```python
from build123d import *

# Parameters (mm, degrees)
BOSS_EXTRUDE1_DEPTH = 2
SKETCH1_3_W         = 10
SKETCH1_3_H         = 4.75
BOSS_EXTRUDE2_DEPTH = 12.7
BOSS_EXTRUDE3_START = 12.7
SKETCH3_W           = 11.9
SKETCH3_H           = 4.75
SKETCH3_W_2         = 10.75
BOSS_EXTRUDE3_DEPTH = 12.7
BOSS_EXTRUDE4_START = 25.4
SKETCH3_3_W         = 11.9
SKETCH3_3_H         = 4.75
SKETCH3_3_W_2       = 10.75
SKETCH3_3_W_3       = 1.15
BOSS_EXTRUDE4_DEPTH = 2
CUT_EXTRUDE1_START  = -1.1
SKETCH2_R           = 1.6
CUT_EXTRUDE1_DEPTH  = 8
CUT_EXTRUDE2_START  = 3.1
SKETCH2_3_R         = 1.6
CUT_EXTRUDE2_DEPTH  = 8
BOSS_EXTRUDE5_START = 10
SKETCH1_4_R         = 2.075
BOSS_EXTRUDE5_DEPTH = 10
FILLET1_R           = 5
CUT_EXTRUDE3_START  = 12.7
SKETCH5_W           = 14.55
SKETCH5_H           = 4.75
CUT_EXTRUDE3_DEPTH  = 2
CUT_EXTRUDE4_START  = 12.7
SKETCH6_W           = 7.7
SKETCH6_H           = 4.75
CUT_EXTRUDE4_DEPTH  = 4


with BuildPart() as part:
    # Sketch1 → Boss-Extrude1 (new body)
    with BuildSketch(Plane(origin=(0, 0, 0), x_dir=(1, 0, 0), z_dir=(0, 1, 0))):
        Polygon((-1.1, 16.25), (-1.1, -16.25), (8.9, -16.25), (8.9, -11.5), (17.65, -11.5), (17.65, 16.25), align=None)
    extrude(amount=-BOSS_EXTRUDE1_DEPTH)

    # Sketch1<3> → Boss-Extrude2 (add)
    with BuildSketch(Plane(origin=(0, 0, 0), x_dir=(1, 0, 0), z_dir=(0, 1, 0))):
        Polygon((6.45, 16.25), (-1.1, 16.25), (-1.1, 11.5), (17.65, 11.5), (17.65, 16.25), align=None)
        with Locations((3.9, -13.875)):
            Rectangle(SKETCH1_3_W, SKETCH1_3_H)
    extrude(amount=BOSS_EXTRUDE2_DEPTH)

    # Sketch3 → Boss-Extrude3 (add)
    with BuildSketch(Plane(origin=(0, 0, 0), x_dir=(1, 0, 0), z_dir=(0, 1, 0)).offset(BOSS_EXTRUDE3_START)):
        with Locations((-2.85, 13.875)):
            Rectangle(SKETCH3_W, SKETCH3_H)
        with Locations((-2.275, -13.875)):
            Rectangle(SKETCH3_W_2, SKETCH3_H)
    extrude(amount=BOSS_EXTRUDE3_DEPTH)

    # Sketch3<3> → Boss-Extrude4 (add)
    with BuildSketch(Plane(origin=(0, 0, 0), x_dir=(1, 0, 0), z_dir=(0, 1, 0)).offset(BOSS_EXTRUDE4_START)):
        with Locations((-2.85, 13.875)):
            Rectangle(SKETCH3_3_W, SKETCH3_3_H)
        Polygon((3.1, -11.5), (3.1, 11.5), (-8.8, 11.5), (-8.8, -11.5), (-7.65, -11.5), align=None)
        with Locations((-2.275, -13.875)):
            Rectangle(SKETCH3_3_W_2, SKETCH3_3_H)
        with Locations((-8.225, -13.875)):
            Rectangle(SKETCH3_3_W_3, SKETCH3_3_H)
    extrude(amount=BOSS_EXTRUDE4_DEPTH)

    # Sketch2 → Cut-Extrude1 (cut)
    with BuildSketch(Plane(origin=(0, 0, 0), x_dir=(0, 0, -1), z_dir=(1, 0, 0)).offset(CUT_EXTRUDE1_START)):
        with Locations(Location((-13.7, 6.45, 0), (0, 0, 180))):
            Circle(SKETCH2_R)
        with Locations(Location((13.7, 6.45, 0), (0, 0, 180))):
            Circle(SKETCH2_R)
    extrude(amount=CUT_EXTRUDE1_DEPTH, mode=Mode.SUBTRACT)

    # Sketch2<3> → Cut-Extrude2 (cut)
    with BuildSketch(Plane(origin=(0, 0, 0), x_dir=(0, 0, -1), z_dir=(1, 0, 0)).offset(CUT_EXTRUDE2_START)):
        with Locations(Location((13.7, 19.15, 0), (0, 0, 180))):
            Circle(SKETCH2_3_R)
        with Locations(Location((-13.7, 19.15, 0), (0, 0, 180))):
            Circle(SKETCH2_3_R)
    extrude(amount=-CUT_EXTRUDE2_DEPTH, mode=Mode.SUBTRACT)

    # Sketch1<4> → Boss-Extrude5 (add)
    # profile 1 of 2: a face of its own
    with BuildSketch(Plane(origin=(0, 0, 0), x_dir=(1, 0, 0), z_dir=(0, 1, 0)).offset(BOSS_EXTRUDE5_START)):
        Polygon((-1.25, 16.25), (-1.1, 16.25), (6.45, 16.25), (6.45, 23.05), (-1.25, 23.05), align=None)
        with Locations(Location((2.6, 19.85, 0), (0, 0, 270))):
            Circle(SKETCH1_4_R, mode=Mode.SUBTRACT)
    # profile 2 of 2: a face of its own
    with BuildSketch(Plane(origin=(0, 0, 0), x_dir=(1, 0, 0), z_dir=(0, 1, 0)).offset(BOSS_EXTRUDE5_START)):
        Polygon((-3.95, -23.05), (-3.95, -16.25), (-8.8, -16.25), (-11.65, -16.25), (-11.65, -23.05), align=None)
        with Locations(Location((-7.8, -19.85, 0), (0, 0, 270))):
            Circle(SKETCH1_4_R, mode=Mode.SUBTRACT)
    extrude(amount=BOSS_EXTRUDE5_DEPTH)

    # Fillet1
    fillet1_edges = [part.edges().sort_by_distance(p)[0] for p in [
        (3.9, -2, 16.25),
        (-2.85, 27.4, 16.25),
        (8.275, -2, -16.25),
        (-2.85, 27.4, -16.25),
    ]]
    fillet(fillet1_edges, radius=FILLET1_R)

    # Sketch5 → Cut-Extrude3 (cut)
    with BuildSketch(Plane(origin=(0, 0, 0), x_dir=(1, 0, 0), z_dir=(0, 1, 0)).offset(CUT_EXTRUDE3_START)):
        with Locations((10.375, 13.875)):
            Rectangle(SKETCH5_W, SKETCH5_H)
    extrude(amount=-CUT_EXTRUDE3_DEPTH, mode=Mode.SUBTRACT)

    # Sketch6 → Cut-Extrude4 (cut)
    with BuildSketch(Plane(origin=(0, 0, 0), x_dir=(1, 0, 0), z_dir=(0, 1, 0)).offset(CUT_EXTRUDE4_START)):
        with Locations((-4.95, 13.875)):
            Rectangle(SKETCH6_W, SKETCH6_H)
    extrude(amount=CUT_EXTRUDE4_DEPTH, mode=Mode.SUBTRACT)


solid = part.part
```
Here's how the part is built. I have some questions about the finished solid (model axes, mm). A direction names the side the tool comes from. Coordinates: 2 decimals unless noted, no trailing zeros. Loops run counter-clockwise (first coordinate to the right, second up) from the corner with the lowest first, then second, coordinate; pieces in that order, holes last. Notation, with made-up numbers: (-21, 64.5) - (22, 64.5) arc R7 ccw to (22, 75.5) - close; hole circle Ø4 at (68.5, -7.5). An arc over 180 degrees is marked (long way). Answer as CSV lines item,"result".
Q1. For pin 1 (15 mm diameter, centred on y = 7, z = 6, fed in from -X); pin 2 (1.5 mm diameter, centred on y = 12.5, z = -13.5, fed in from +X); pin 3 (2.5 mm diameter, centred on x = 5, y = 16, fed in from +Z); pin 4 (5 mm diameter, centred on y = 15.5, z = -7, fed in from +X), each with a flat end and sliding along its axis, tell me the tip position at first contact or that it passes through.
Response:
pin 1,"x = -1.1"
pin 2,"x = 3.1"
pin 3,"z = -16.25"
pin 4,"through"
Q2. If I drill on L1, parallel to Z at x = 4, y = 6.45; L2, parallel to X at y = 16.5, z = 19.85 (3 decimals); L3, parallel to X at y = 16, z = -19.85 (3 decimals), over which ranges is the centre line in solid material (lowest first)? Write a range as [from, to].
Response:
L1,"[-16.25, -15.3], [-12.1, -11.5], [11.5, 12.1], [15.3, 16.25]"
L2,"[-11.65, -9.875], [-5.725, -3.95]"
L3,"[-1.25, 0.525], [4.675, 6.45]"
Q3. For faces 4 (the face through (-1.25, 15, -20)), 5 (the face through (3, 10, -17)), 6 (the face through (6.9, 6, 14)), 7 (the face through (-7.65, 19, 14)), 8 (the face through (6.45, 15, -20)), which set-ups out of +Z, -Z, +X, -X, +Y, -Y let a thin tool reach every point of the face, with its end or its side?
Response:
face 4,"-Z, -X, +Y, -Y"
face 5,"-Z, +X, -X, -Y"
face 6,"-X"
face 7,"-X, -Y"
face 8,"-Z, +X, +Y, -Y"
Q4. We'd pull the mould along Z, two halves only. Please class faces 1 (the face through (-4, 12.7, 14)), 2 (the face through (1, 13, 11.5)), 3 (the face through (4.24, -0.57, 14.75)): pulls with the +Z half, pulls with the -Z half, needs draft (parallel to the pull), parting line crosses it, or undercut.
Response:
face 1,"needs draft"
face 2,"undercut"
face 3,"pulls with the +Z half"
Q5. If we section it at B-B, the plane y = 11.25: Write out the boundary of the cut face in (x, z) (3 decimals).
Response:
outline,"(-11.65, 16.25) - (-3.95, 16.25) - (-3.95, 23.05) - (-11.65, 23.05) - close; (-1.25, -23.05) - (6.45, -23.05) - (6.45, -16.25) - (3.1, -16.25) - (3.1, -11.5) - (-1.1, -11.5) - (-1.1, -16.25) - (-1.25, -16.25) - close; (-1.1, 11.5) - (8.9, 11.5) - (8.9, 16.25) - (-1.1, 16.25) - close; hole circle Ø4.15 at (-7.8, 19.85); hole circle Ø4.15 at (2.6, -19.85)"
Q6. If we section it at C-C, the plane y = 4: Write out the boundary of the cut face in (x, z).
Response:
outline,"(-1.1, -16.25) - (17.65, -16.25) - (17.65, -11.5) - (-1.1, -11.5) - close; (-1.1, 11.5) - (8.9, 11.5) - (8.9, 16.25) - (-1.1, 16.25) - close"
Q7. If we section it at A-A, the plane x = 2.6: Write out the boundary of the cut face in (y, z) (3 decimals).
Response:
outline,"(-2, -11.25) arc R5 ccw to (3, -16.25) - (10, -16.25) - (10, -17.775) - (20, -17.775) - (20, -16.25) - (22.4, -16.25) arc R5 ccw to (27.4, -11.25) - (27.4, 11.25) arc R5 ccw to (22.4, 16.25) - (3, 16.25) arc R5 ccw to (-2, 11.25) - close; (10, -23.05) - (20, -23.05) - (20, -21.925) - (10, -21.925) - close; hole (0, -11.5) - (25.4, -11.5) - (25.4, 11.5) - (0, 11.5) - close; hole circle Ø3.2 at (6.45, -13.7); hole circle Ø3.2 at (6.45, 13.7); hole circle Ø3.2 at (19.15, -13.7); hole circle Ø3.2 at (19.15, 13.7)"
Q8. If we section it at D-D, the plane x = -2.5: Write out the boundary of the cut face in (y, z), and give its area (3 significant figures).
Response:
outline,"(12.7, 11.5) - (25.4, 11.5) - (25.4, -11.5) - (16.7, -11.5) - (16.7, -16.25) - (22.4, -16.25) arc R5 ccw to (27.4, -11.25) - (27.4, 11.25) arc R5 ccw to (22.4, 16.25) - (12.7, 16.25) - close; hole circle Ø3.2 at (19.15, -13.7); hole circle Ø3.2 at (19.15, 13.7)"
area,"140 mm2"
